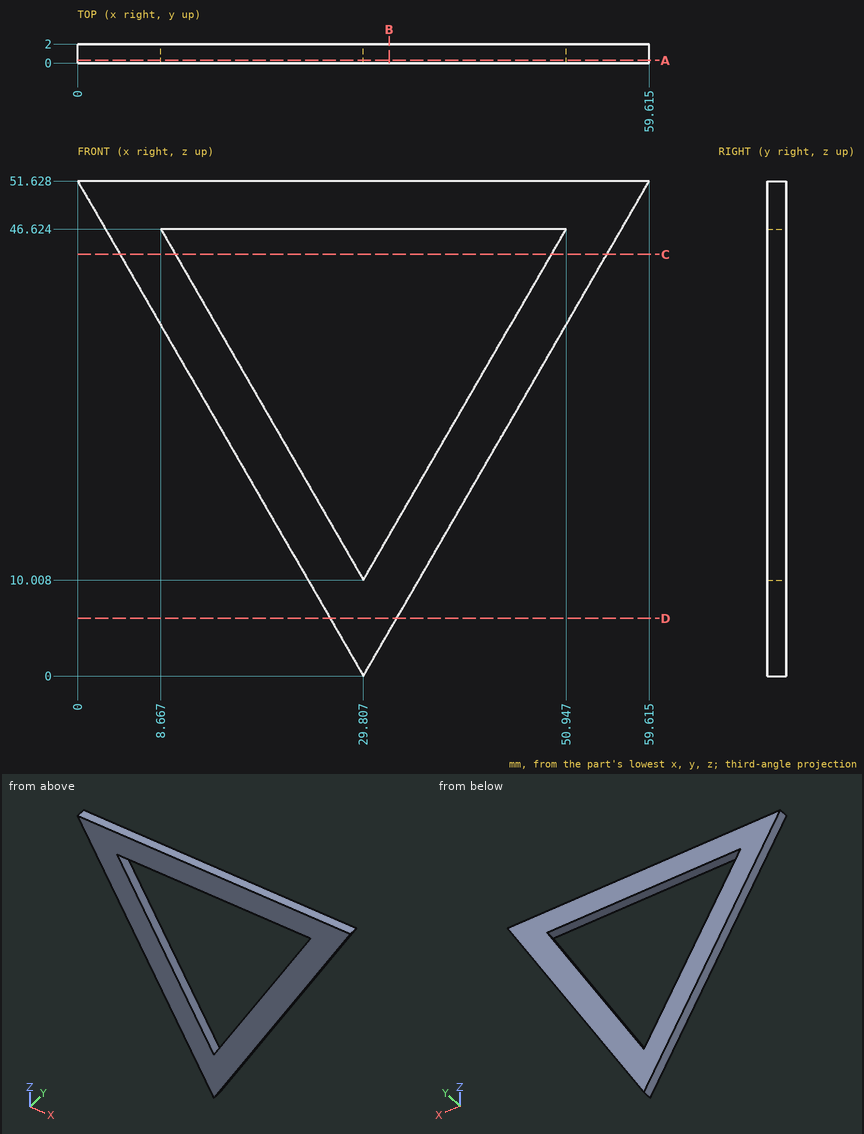
Study the drawing (mm; zero at the part's minimum x, y, z) and answer. Round coordinates to 2 decimals unless told otherwise and drop trailing zeros. Loops run counter-clockwise (first coordinate to the right, second up) from the corner with the lowest first, then second, coordinate; pieces in that order, holes last. Notation, with made-up numbers: (-17.75, -8.5) - (34.25, -8.5) arc R15 cw to (34.25, 0.5) - close; hole circle Ø6 at (-4, 33.5). An arc over 180 degrees is marked (long way). Use one line per item in the form item = value. Start each with the question number.
1. The part is cut by section B-B on x = 32.5. Determine the outline of the cut face in (y, z).
2. The part is cut by section D-D on z = 6. Determine the outline of the cut face in (x, y).
3. Consider line 1 (Z direction, x = 49.5, y = 1.5) (1 decimal); line 2 (Z direction, x = 21, y = 0.15) (1 decimal); line 3 (X direction, y = 0.5, z = 19) (1 decimal). Determine where each line is inside the solid, lowest interval first. Write a range as [from, to].
4. The part is cut by section A-A on y = 0.3. Determine the outline of the cut face in (x, z) (1 decimal).
5. Given pin 1 Ø0.6 at (x, y) = (21, 1.5) entering from -Z (1 decimal), flat-ended and moving along its own axis, determine where the tip first touches the part or whether it passes through.
6. The part is cut by section C-C on z = 44. Determine the outline of the cut face in (x, y), then the cut area to 3 significant figures.
Geometry check:
q1.outline = (0, 4.66) - (2, 4.66) - (2, 14.67) - (0, 14.67) - close; (0, 46.62) - (2, 46.62) - (2, 51.63) - (0, 51.63) - close
q2.outline = (26.34, 0) - (33.27, 0) - (33.27, 2) - (26.34, 2) - close
q3.line_1 = [34.1, 44.1], [46.6, 51.6]
q3.line_2 = [15.3, 25.3], [46.6, 51.6]
q3.line_3 = [18.8, 24.6], [35, 40.8]
q4.outline = (0, 51.6) - (29.8, 0) - (59.6, 51.6) - close; hole (8.7, 46.6) - (29.8, 10) - (50.9, 46.6) - close
q5.pin_1 = 14.7
q6.outline = (4.4, 0) - (10.18, 0) - (10.18, 2) - (4.4, 2) - close; (49.43, 0) - (55.21, 0) - (55.21, 2) - (49.43, 2) - close
q6.area = 23.1 mm^2
